Source: CAD feature listing. Evaluate the final solid. Frame: model axes, mm. Round coordinates to 2 decimals unless told otherwise and drop trailing zeros. Order: outer loops, then holes, each group sorted by start corner. A loop starts at its lowest first (then second) coordinate and runs counter-clockwise, first axis right, second up.
```python
from build123d import *

# Parameters (mm, degrees)
SKETCH1_R           = 9
SKETCH1_R_2         = 3
SKETCH1_R_3         = 1.65
BOSS_EXTRUDE1_DEPTH = 6.35
CUT_EXTRUDE1_DEPTH  = 10


with BuildPart() as part:
    # Sketch1 → Boss-Extrude1 (new body)
    with BuildSketch(Plane.XY):
        with BuildLine():
            Line((-15, 15), (-15, -15))
            ThreePointArc((-15, -15), (-14.275727836, -25.159324804), (-12.117561222, -35.113156605))
            ThreePointArc((-12.117561222, -35.113156605), (-11.640196728, -62.923473964), (-25.409366876, -87.090633124))
            ThreePointArc((-25.409366876, -87.090633124), (-27.067678424, -89.572471742), (-27.65, -92.5))
            Line((-27.65, -92.5), (-27.65, -97))
            ThreePointArc((-27.65, -97), (-26.771320344, -99.121320344), (-24.65, -100))
            Line((-24.65, -100), (24.65, -100))
            ThreePointArc((24.65, -100), (26.771320344, -99.121320344), (27.65, -97))
            Line((27.65, -97), (27.65, -92.5))
            ThreePointArc((27.65, -92.5), (27.067678424, -89.572471742), (25.409366876, -87.090633124))
            ThreePointArc((25.409366876, -87.090633124), (11.640196728, -62.923473964), (12.117561222, -35.113156605))
            ThreePointArc((12.117561222, -35.113156605), (14.275727836, -25.159324804), (15, -15))
            Line((15, -15), (15, 15))
            ThreePointArc((15, 15), (14.275727836, 25.159324804), (12.117561222, 35.113156605))
            ThreePointArc((12.117561222, 35.113156605), (11.640196728, 62.923473964), (25.409366876, 87.090633124))
            ThreePointArc((25.409366876, 87.090633124), (27.067678424, 89.572471742), (27.65, 92.5))
            Line((27.65, 92.5), (27.65, 97))
            ThreePointArc((27.65, 97), (26.771320344, 99.121320344), (24.65, 100))
            Line((24.65, 100), (-24.65, 100))
            ThreePointArc((-24.65, 100), (-26.771320344, 99.121320344), (-27.65, 97))
            Line((-27.65, 97), (-27.65, 92.5))
            ThreePointArc((-27.65, 92.5), (-27.067678424, 89.572471742), (-25.409366876, 87.090633124))
            ThreePointArc((-25.409366876, 87.090633124), (-11.640196728, 62.923473964), (-12.117561222, 35.113156605))
            ThreePointArc((-12.117561222, 35.113156605), (-14.275727836, 25.159324804), (-15, 15))
        make_face()
        Circle(SKETCH1_R, mode=Mode.SUBTRACT)
        with Locations((0, 44.9961)):
            Circle(SKETCH1_R_2, mode=Mode.SUBTRACT)
        with Locations((20, 92.5)):
            Circle(SKETCH1_R_3, mode=Mode.SUBTRACT)
        with Locations((-20, 92.5)):
            Circle(SKETCH1_R_3, mode=Mode.SUBTRACT)
        with Locations((-20, -92.5)):
            Circle(SKETCH1_R_3, mode=Mode.SUBTRACT)
        with Locations((20, -92.5)):
            Circle(SKETCH1_R_3, mode=Mode.SUBTRACT)
        with BuildLine():
            Line((3, -43.0351625), (3, -46.9570375))
            ThreePointArc((3, -46.9570375), (0, -49.9570375), (-3, -46.9570375))
            Line((-3, -46.9570375), (-3, -43.0351625))
            ThreePointArc((-3, -43.0351625), (0, -40.0351625), (3, -43.0351625))
        make_face(mode=Mode.SUBTRACT)
    extrude(amount=BOSS_EXTRUDE1_DEPTH)

    # Sketch3 → Cut-Extrude1 (cut)
    with BuildSketch(Plane.XY.offset(6.35)):
        with BuildLine():
            Line((-8.5, 101), (-8.5, 86))
            ThreePointArc((-8.5, 86), (-7.914213562, 84.585786438), (-6.5, 84))
            Line((-6.5, 84), (6.5, 84))
            ThreePointArc((6.5, 84), (7.914213562, 84.585786438), (8.5, 86))
            Line((8.5, 86), (8.5, 101))
            Line((8.5, 101), (-8.5, 101))
        make_face()
    extrude(amount=-CUT_EXTRUDE1_DEPTH, mode=Mode.SUBTRACT)


solid = part.part
```
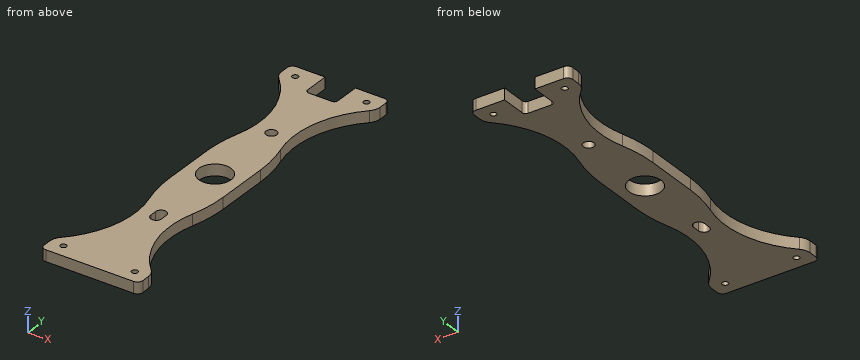
1. Section B-B on z = 1. State how many separate pieces and enclosed holes the cut face has, plus the area to 3 significant figures.
2. Section C-C on y = 21. Return loops of the section in (x, z).
3. First-contact query: pin 1 (3 mm diameter, centred on y = 90, z = 3.5, fed in from +X); pin 2 (2 mm diameter, centred on y = 56.5, z = 2, fed in from -X); pin 3 (3 mm diameter, centred on y = -7.5, z = 1.5, fed in from +X). Flat tips, straight axial feed; report the tip coordinate or a pass-through.
4. Line query: line 1 along Y through (x, z) = (0, 4); line 2 along Y through (x, z) = (0.5, 3); line 3 along X through (y, z) = (92.5, 3.25). Output: solid intervals per line, ascending.
5. Section D-D on y = -26.5. Return loops of the section in (x, z).
6. Section A-A on y = 0. Return loops of the section in (x, z), plus the area to 3 significant figures.
Result:
1. separate pieces: 1
1. enclosed holes: 7
1. area: 5,630 mm2
2. outline: (-14.75, 0) - (14.75, 0) - (14.75, 6.35) - (-14.75, 6.35) - close
3. pin 1: stops at x = 27.58
3. pin 2: stops at x = -10.55
3. pin 3: stops at x = 15
4. line 1: y = -100 to -49.96, -40.04 to -9, 9 to 42, 48 to 84
4. line 2: y = -100 to -49.92, -40.08 to -8.99, 8.99 to 42.04, 47.95 to 84
4. line 3: x = -27.65 to -21.65, -18.35 to -8.5, 8.5 to 18.35, 21.65 to 27.65
5. outline: (-14.07, 0) - (14.07, 0) - (14.07, 6.35) - (-14.07, 6.35) - close
6. outline: (-15, 0) - (-9, 0) - (-9, 6.35) - (-15, 6.35) - close; (9, 0) - (15, 0) - (15, 6.35) - (9, 6.35) - close
6. area: 76.2 mm2
